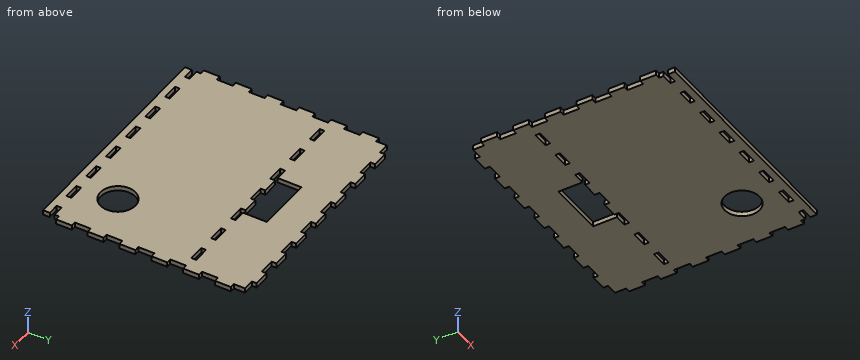
```python
from build123d import *

# Parameters (mm, degrees)
CROQUIS1_W              = 10
CROQUIS1_H              = 3
CROQUIS1_R              = 11
SALIENTE_EXTRUIR1_DEPTH = 3


with BuildPart() as part:
    # Croquis1 → Saliente-Extruir1 (new body)
    with BuildSketch(Plane.XY):
        Polygon((-35, 71.5), (-45, 71.5), (-45, 68.5), (-55, 68.5), (-55, 71.5), (-65, 71.5), (-65, 68.5), (-72, 68.5), (-72, 61.5), (-75, 61.5), (-75, 51.5), (-72, 51.5), (-72, 41.5), (-75, 41.5), (-75, 31.5), (-72, 31.5), (-72, 21.5), (-75, 21.5), (-75, 11.5), (-72, 11.5), (-72, 1.5), (-75, 1.5), (-75, -8.5), (-72, -8.5), (-72, -18.5), (-75, -18.5), (-75, -28.5), (-72, -28.5), (-72, -38.5), (-75, -38.5), (-75, -48.5), (-72, -48.5), (-72, -51.25), (-65, -51.25), (-65, -54.25), (-72, -54.25), (-72, -58.5), (72, -58.5), (72, -54.25), (65, -54.25), (65, -51.25), (72, -51.25), (72, -48.5), (75, -48.5), (75, -38.5), (72, -38.5), (72, -28.5), (75, -28.5), (75, -18.5), (72, -18.5), (72, -8.5), (75, -8.5), (75, 1.5), (72, 1.5), (72, 11.5), (75, 11.5), (75, 21.5), (72, 21.5), (72, 31.5), (75, 31.5), (75, 41.5), (72, 41.5), (72, 51.5), (75, 51.5), (75, 61.5), (72, 61.5), (72, 68.5), (65, 68.5), (65, 71.5), (55, 71.5), (55, 68.5), (45, 68.5), (45, 71.5), (35, 71.5), (35, 68.5), (25, 68.5), (25, 71.5), (15, 71.5), (15, 68.5), (5, 68.5), (5, 71.5), (-5, 71.5), (-5, 68.5), (-15, 68.5), (-15, 71.5), (-25, 71.5), (-25, 68.5), (-35, 68.5), align=None)
        with Locations((-50, -52.75)):
            Rectangle(CROQUIS1_W, CROQUIS1_H, mode=Mode.SUBTRACT)
        with Locations((-30, -52.75)):
            Rectangle(CROQUIS1_W, CROQUIS1_H, mode=Mode.SUBTRACT)
        with Locations((-10, -52.75)):
            Rectangle(CROQUIS1_W, CROQUIS1_H, mode=Mode.SUBTRACT)
        with Locations((10, -52.75)):
            Rectangle(CROQUIS1_W, CROQUIS1_H, mode=Mode.SUBTRACT)
        with Locations((30, -52.75)):
            Rectangle(CROQUIS1_W, CROQUIS1_H, mode=Mode.SUBTRACT)
        with Locations((50, -52.75)):
            Rectangle(CROQUIS1_W, CROQUIS1_H, mode=Mode.SUBTRACT)
        with Locations((42.725871833, -29.529627422)):
            Circle(CROQUIS1_R, mode=Mode.SUBTRACT)
        with Locations((-60, 32)):
            Rectangle(CROQUIS1_W, CROQUIS1_H, mode=Mode.SUBTRACT)
        with Locations((-40, 32)):
            Rectangle(CROQUIS1_W, CROQUIS1_H, mode=Mode.SUBTRACT)
        Polygon((-25, 30.5), (-25, 33.5), (-17.5, 33.5), (-17.5, 48.5), (17.5, 48.5), (17.5, 33.5), (25, 33.5), (25, 30.5), (15, 30.5), (15, 33.5), (5, 33.5), (5, 30.5), (-5, 30.5), (-5, 33.5), (-15, 33.5), (-15, 30.5), align=None, mode=Mode.SUBTRACT)
        with Locations((40, 32)):
            Rectangle(CROQUIS1_W, CROQUIS1_H, mode=Mode.SUBTRACT)
        with Locations((60, 32)):
            Rectangle(CROQUIS1_W, CROQUIS1_H, mode=Mode.SUBTRACT)
    extrude(amount=SALIENTE_EXTRUIR1_DEPTH)


solid = part.part
```
The model under review builds one solid part; all positions refer to its coordinate system, in mm. Round coordinates to 2 decimals unless told otherwise and drop trailing zeros. Order: outer loops, then holes, each group sorted by start corner. A loop starts at its lowest first (then second) coordinate and runs counter-clockwise, first axis right, second up. Notation, with made-up numbers: (8.5, 88.5) - (39.5, 88.5) arc R10 cw to (39.5, 99.5) - close; hole circle Ø11 at (-28.5, 78). An arc over 180 degrees is marked (long way). Answer in a Markdown table with one row per item.
(1) Take a section at C-C on y = -34.5. Write out the cut boundary in (x, z).
Result set:
| item | result |
|---|---|
| outline | (-72, 0) - (32.91, 0) - (32.91, 3) - (-72, 3) - close; (52.54, 0) - (72, 0) - (72, 3) - (52.54, 3) - close |
(2) Clearance check with flat-ended pins moving along their axes: P1, Ø1.5, axis at x = 73.5, z = 1.5, coming from the +Y side; P2, Ø1.5, axis at y = -33.5, z = 1.5, coming from the +X side; P3, Ø1.5, axis at y = 44, z = 0.5, coming from the -X side. State where each tip first meets the part, or that it passes through.
Result set:
| item | result |
|---|---|
| P1 | stops at y = 61.5 |
| P2 | stops at x = 72 |
| P3 | stops at x = -72 |
(3) Take a section at B-B on x = 39. Write out the cut boundary in (y, z), plus the area to 3 significant figures.
Result set:
| item | result |
|---|---|
| outline | (-58.5, 0) - (-39.88, 0) - (-39.88, 3) - (-58.5, 3) - close; (-19.18, 0) - (30.5, 0) - (30.5, 3) - (-19.18, 3) - close; (33.5, 0) - (71.5, 0) - (71.5, 3) - (33.5, 3) - close |
| area | 319 mm2 |
(4) For line 1 (Y direction, x = 11.5, z = 2.55); line 2 (Y direction, x = -36, z = 1.3); line 3 (Y direction, x = 33, z = 0.7), list the stretches that pass through material, from the lowest coordinate up. Write a range as from..to.
Result set:
| item | result |
|---|---|
| line 1 | y = -58.5..-54.25, -51.25..33.5, 48.5..68.5 |
| line 2 | y = -58.5..30.5, 33.5..71.5 |
| line 3 | y = -58.5..-54.25, -51.25..-34.67, -24.39..68.5 |
(5) Take a section at D-D on y = 8. Write out the cut boundary in (x, z).
Result set:
| item | result |
|---|---|
| outline | (-72, 0) - (72, 0) - (72, 3) - (-72, 3) - close |
(6) Take a section at A-A on x = 2.5. Write out the cut boundary in (y, z).
Result set:
| item | result |
|---|---|
| outline | (-58.5, 0) - (30.5, 0) - (30.5, 3) - (-58.5, 3) - close; (48.5, 0) - (71.5, 0) - (71.5, 3) - (48.5, 3) - close |
